Work out the finished part from the listing and answer in its coordinate system (mm). Face numbers are marked on the shaded views. Round coordinates to 2 decimals unless told otherwise and drop trailing zeros. Loops run counter-clockwise (first coordinate to the right, second up) from the corner with the lowest first, then second, coordinate; pieces in that order, holes last. Notation, with made-up numbers: M 32.5,-15 L 87.5,-15 A18 ccw 87.5,12 Z; hole C 4.25,52 d3. An arc over 180 degrees is marked long. One line per item, written item: value.
```python
from build123d import *

# Parameters (mm, degrees)
SKETCH1_W           = 50
SKETCH1_H           = 50
SKETCH1_R           = 1.3
BOSS_EXTRUDE1_DEPTH = 6
FILLET1_R           = 8
SKETCH2_W           = 4
SKETCH2_H           = 8
BOSS_EXTRUDE2_DEPTH = 6
FILLET2_R           = 4
SKETCH6_R           = 1.6
CUT_EXTRUDE3_DEPTH  = 36
SKETCH4_W           = 5
SKETCH4_H           = 8
BOSS_EXTRUDE4_DEPTH = 5
FILLET3_R           = 3.5
SKETCH5_R           = 0.7
CUT_EXTRUDE2_DEPTH  = 44
CHAMFER3_SIZE       = 1.2


with BuildPart() as part:
    # Sketch1 → Boss-Extrude1 (new body)
    with BuildSketch(Plane(origin=(0, 0, 0), x_dir=(0, 0, -1), z_dir=(1, 0, 0))):
        Rectangle(SKETCH1_W, SKETCH1_H)
        with Locations((-15, 15)):
            Circle(SKETCH1_R, mode=Mode.SUBTRACT)
        with Locations((15, 15)):
            Circle(SKETCH1_R, mode=Mode.SUBTRACT)
        with Locations((15, -15)):
            Circle(SKETCH1_R, mode=Mode.SUBTRACT)
        with Locations((-15, -15)):
            Circle(SKETCH1_R, mode=Mode.SUBTRACT)
    extrude(amount=BOSS_EXTRUDE1_DEPTH)

    # Fillet1
    fillet1_edges = [part.edges().sort_by_distance(p)[0] for p in [
        (3, -25, -25),
        (3, -25, 25),
        (3, 25, 25),
        (3, 25, -25),
    ]]
    fillet(fillet1_edges, radius=FILLET1_R)

    # Sketch2 → Boss-Extrude2 (add)
    with BuildSketch(Plane.ZY):
        with Locations((-5.05, -21)):
            Rectangle(SKETCH2_W, SKETCH2_H)
        with Locations((5.05, -21)):
            Rectangle(SKETCH2_W, SKETCH2_H)
    extrude(amount=BOSS_EXTRUDE2_DEPTH)

    # Fillet2
    fillet2_edges = [part.edges().sort_by_distance(p)[0] for p in [
        (-6, -25, 5.05),
        (-6, -25, -5.05),
        (-6, -17, -5.05),
        (-6, -17, 5.05),
    ]]
    fillet(fillet2_edges, radius=FILLET2_R - 0.0001)  # a hair under: the kernel refuses the full size

    # Sketch6 → Cut-Extrude3 (cut)
    with BuildSketch(Plane(origin=(0, 0, -7.05), x_dir=(-1, 0, 0), z_dir=(0, 0, -1))):
        with Locations((3, -21)):
            Circle(SKETCH6_R)
    extrude(amount=-CUT_EXTRUDE3_DEPTH, mode=Mode.SUBTRACT)

    # Sketch4 → Boss-Extrude4 (add)
    with BuildSketch(Plane.ZY):
        with Locations((-17.5, -9)):
            Rectangle(SKETCH4_W, SKETCH4_H)
        with Locations((17.5, -9)):
            Rectangle(SKETCH4_W, SKETCH4_H)
    extrude(amount=BOSS_EXTRUDE4_DEPTH)

    # Fillet3
    fillet3_edges = [part.edges().sort_by_distance(p)[0] for p in [
        (-5, -5, -17.5),
        (-5, -13, -17.5),
        (-5, -13, 17.5),
        (-5, -5, 17.5),
    ]]
    fillet(fillet3_edges, radius=FILLET3_R)

    # Sketch5 → Cut-Extrude2 (cut)
    with BuildSketch(Plane(origin=(0, 0, -20), x_dir=(-1, 0, 0), z_dir=(0, 0, -1))):
        with Locations(Location((2.5, -9, 0), (0, 0, 90))):
            Circle(SKETCH5_R)
    extrude(amount=-CUT_EXTRUDE2_DEPTH, mode=Mode.SUBTRACT)

    # Chamfer3
    chamfer3_edges = [part.edges().sort_by_distance(p)[0] for p in [
        (-5, -9, 15),
        (-0.75, -13, 15),
        (-0.75, -5, 15),
        (-3.974873734, -6.025126266, 15),
        (-3.974873734, -11.974873734, 15),
        (-5, -9, -15),
        (-0.75, -5, -15),
        (-0.75, -13, -15),
        (-3.974873734, -6.025126266, -15),
        (-3.974873734, -11.974873734, -15),
    ]]
    chamfer(chamfer3_edges, length=CHAMFER3_SIZE)


solid = part.part
```
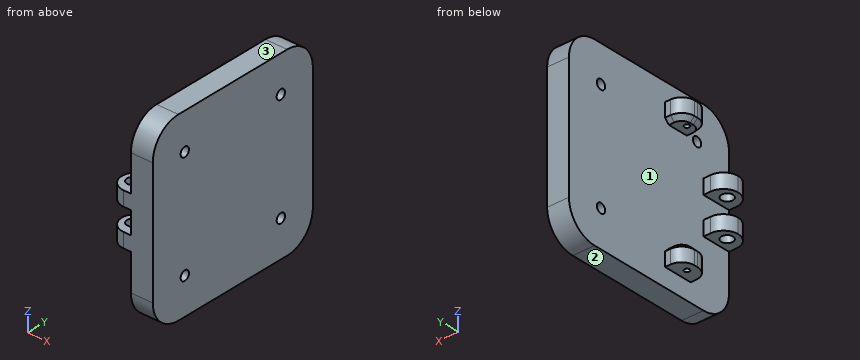
1) Find the intervals of material crossed by probe 1 along Y at (x, z) = (1.75, 15); probe 2 along X at (y, z) = (-9, -18.6); probe 3 along Y at (x, z) = (2.75, -14), in increasing order. Write a range as from..to.
Check values:
probe 1: -25..-16.3, -13.7..13.7, 16.3..25
probe 2: -5..-3.2, -1.8..6
probe 3: -25..-15.83, -14.17..14.17, 15.83..25
2) Find section A-A (y = -15). Give the vertices of the cut face in (x, z).
Check values:
outline: M 0,-25 L 6,-25 L 6,-16.3 L 0,-16.3 Z; M 0,-13.7 L 6,-13.7 L 6,13.7 L 0,13.7 Z; M 0,16.3 L 6,16.3 L 6,25 L 0,25 Z
3) Each of these flat-tipped pins is pushed along its axis until it touches: pin 1 (1.5 mm diameter, centred on x = 3, y = -19, fed in from -Z); pin 2 (1.7 mm diameter, centred on x = -0.5, z = -19, fed in from +Y); pin 3 (2 mm diameter, centred on y = -13.5, z = 10.5, fed in from -X). Where does it stop, or does it pass through?
Check values:
pin 1: z = -24.9
pin 2: y = 24.89
pin 3: x = 0
4) Find section B-B (y = 12.5). Give the vertices of the cut face in (x, z), then the cut area to 3 significant figures.
Check values:
outline: M 0,-25 L 6,-25 L 6,25 L 0,25 Z
area: 300 mm2
5) The mould has two halves that part along Z. Classify the marked faces 1, 2 and 3: +Z half, -Z half, draft (parallel to the pull), parting line (faces both ways), or undercut.
Check values:
face 1: undercut
face 2: -Z half
face 3: +Z half
